Build history of the part. All positions in model axes, mm. A direction names the side the tool comes from. Give positions to 0.01 mm unless a question says otherwise; leave off trailing zeros. Write each loop counter-clockwise with the first axis right and the second up, starting at its lowest first coordinate (ties: lowest second). Pieces come first, ordered by that corner, then holes. Notation, with made-up numbers: (-0.5, 10) -> (9.5, 10) arc R15 ccw to (9.5, 16) -> close; hole circle Ø5 at (-22, 29.25). An arc over 180 degrees is marked (long way). Put each result on its own line as item: value.
from build123d import *

# Parameters (mm, degrees)
SKETCH1_W             = 120
SKETCH1_H             = 31.25
BOSS_EXTRUDE1_DEPTH   = 25
SKETCH2_W             = 18.75
SKETCH2_H             = 17.5
CUT_EXTRUDE1_DEPTH    = 124.568364175
F_4_0MM_DOWEL_HOLE1_D = 4
SKETCH5_W             = 120
SKETCH5_H             = 25
BOSS_EXTRUDE2_DEPTH   = 10
SKETCH6_W             = 80
SKETCH6_H             = 6
CUT_EXTRUDE2_DEPTH    = 17.5
FILLET1_R             = 10
SKETCH7_W             = 25
SKETCH7_H             = 18.75
CUT_EXTRUDE3_DEPTH    = 25


with BuildPart() as part:
    # Sketch1 → Boss-Extrude1 (new body)
    with BuildSketch(Plane(origin=(0, 0, 0), x_dir=(1, 0, 0), z_dir=(0, 1, 0))):
        Rectangle(SKETCH1_W, SKETCH1_H)
    extrude(amount=BOSS_EXTRUDE1_DEPTH)

    # Sketch2 → Cut-Extrude1 (cut, through all)
    with BuildSketch(Plane(origin=(60, 0, 0), x_dir=(0, 0, -1), z_dir=(1, 0, 0))):
        with Locations((6.25, 16.25)):
            Rectangle(SKETCH2_W, SKETCH2_H)
    extrude(amount=-CUT_EXTRUDE1_DEPTH, mode=Mode.SUBTRACT)

    # Ø4.0mm Dowel Hole1 (through all)
    with Locations(Plane(origin=(0, 25, 0), x_dir=(1, 0, 0), z_dir=(0, 1, 0))):
        with Locations((50, -9.375), (-50, -9.375)):
            Hole(F_4_0MM_DOWEL_HOLE1_D / 2)

    # Sketch5 → Boss-Extrude2 (add)
    with BuildSketch(Plane.XY.offset(15.625)):
        with Locations((0, 12.5)):
            Rectangle(SKETCH5_W, SKETCH5_H)
    extrude(amount=BOSS_EXTRUDE2_DEPTH)

    # Sketch6 → Cut-Extrude2 (cut)
    with BuildSketch(Plane(origin=(0, 25, 0), x_dir=(1, 0, 0), z_dir=(0, 1, 0))):
        with Locations((0, -9.375)):
            Rectangle(SKETCH6_W, SKETCH6_H)
    extrude(amount=-CUT_EXTRUDE2_DEPTH, mode=Mode.SUBTRACT)

    # Fillet1
    fillet1_edges = [part.edges().sort_by_distance(p)[0] for p in [
        (-60, 12.5, 25.625),
        (60, 12.5, 25.625),
    ]]
    fillet(fillet1_edges, radius=FILLET1_R)

    # Sketch7 → Cut-Extrude3 (cut)
    with BuildSketch(Plane(origin=(0, 7.5, 0), x_dir=(1, 0, 0), z_dir=(0, 1, 0))):
        with Locations((-47.5, 6.25)):
            Rectangle(SKETCH7_W, SKETCH7_H)
        with Locations((47.5, 6.25)):
            Rectangle(SKETCH7_W, SKETCH7_H)
    extrude(amount=-CUT_EXTRUDE3_DEPTH, mode=Mode.SUBTRACT)


solid = part.part
1) Slice it at A-A (x = -17.5). Write the cut outline in (y, z) (3 decimals).
Filled sheet:
outline: (0, -15.625) -> (7.5, -15.625) -> (7.5, 3.125) -> (25, 3.125) -> (25, 6.375) -> (7.5, 6.375) -> (7.5, 12.375) -> (25, 12.375) -> (25, 25.625) -> (0, 25.625) -> close
2) Pin check, flat tips, straight feed: pin 1 (2 mm diameter, centred on y = 2.5, z = -3, fed in from +X); pin 2 (5 mm diameter, centred on x = -12, z = -7.5, fed in from +Y); pin 3 (2 mm diameter, centred on x = 21.5, y = 16, fed in from -Z) (3 decimals); pin 4 (2.5 mm diameter, centred on x = -50, z = 9.375, fed in from +Y). Stop position of each tip, or through.
Filled sheet:
pin 1: x = 35
pin 2: y = 7.5
pin 3: z = 3.125
pin 4: through
3) Slice it at B-B (y = 11.5). Write the cut outline in (x, z) (3 decimals).
Filled sheet:
outline: (-60, 3.125) -> (60, 3.125) -> (60, 15.625) arc R10 ccw to (50, 25.625) -> (-50, 25.625) arc R10 ccw to (-60, 15.625) -> close; hole circle Ø4 at (-50, 9.375); hole (-40, 6.375) -> (40, 6.375) -> (40, 12.375) -> (-40, 12.375) -> close; hole circle Ø4 at (50, 9.375)
4) Tool access for faces 5 (the flat face through (35, 4, -6)), 6 (the flat face through (0, 7.5, -6)), 7 (the flat face through (-1, 16, 12.375)), 8 (the flat face through (-35, 4, -6)): list every direction of +Z, -Z, +X, -X, +Y, -Y with a clear straight run to the whole face (end or side of a thin tool).
Filled sheet:
face 5: -Z, +X, +Y, -Y
face 6: -Z, +X, -X, +Y
face 7: +Y
face 8: -Z, -X, +Y, -Y
5) Slice it at C-C (y = 6). Write the cut outline in (x, z) (3 decimals).
Filled sheet:
outline: (-60, 3.125) -> (-35, 3.125) -> (-35, -15.625) -> (35, -15.625) -> (35, 3.125) -> (60, 3.125) -> (60, 15.625) arc R10 ccw to (50, 25.625) -> (-50, 25.625) arc R10 ccw to (-60, 15.625) -> close; hole circle Ø4 at (-50, 9.375); hole circle Ø4 at (50, 9.375)
6) Wall check: L1, parallel to Z at x = -17, y = 19.25 (3 decimals); L2, parallel to Z at x = -50, y = 11 (3 decimals); L3, parallel to X at y = 15.75, z = 11. Give the ranges that are in metal, low to high.
Filled sheet:
L1: 3.125 to 6.375, 12.375 to 25.625
L2: 3.125 to 7.375, 11.375 to 25.625
L3: -60 to -51.17, -48.83 to -40, 40 to 48.83, 51.17 to 60
7) Pull direction X, two halves, no side cores. Call faces 1 (the flat face through (-1, 7.5, 9)), 2 (the flat face through (40, 16, 9)), 3 (the flat face through (60, 12, 9)), 4 (the flat face through (-1, 0, 9)): released by +X, released by -X, zero draft, split by the parting line, or undercut.
Filled sheet:
face 1: undercut
face 2: undercut
face 3: released by +X
face 4: zero draft
